Part print with two shaded views. Sizes in mm from the minimum x, y, z corner. Give positions to 0.01 mm unless a question says otherwise; leave off trailing zeros. Loops run counter-clockwise (first coordinate to the right, second up) from the corner with the lowest first, then second, coordinate; pieces in that order, holes last. Notation, with made-up numbers: M 41,-8 L 71,-8 A14 ccw 71,-4 Z; hole C -33,-30.5 d9. An arc over 180 degrees is marked long. Answer in a Markdown table with one row per item.
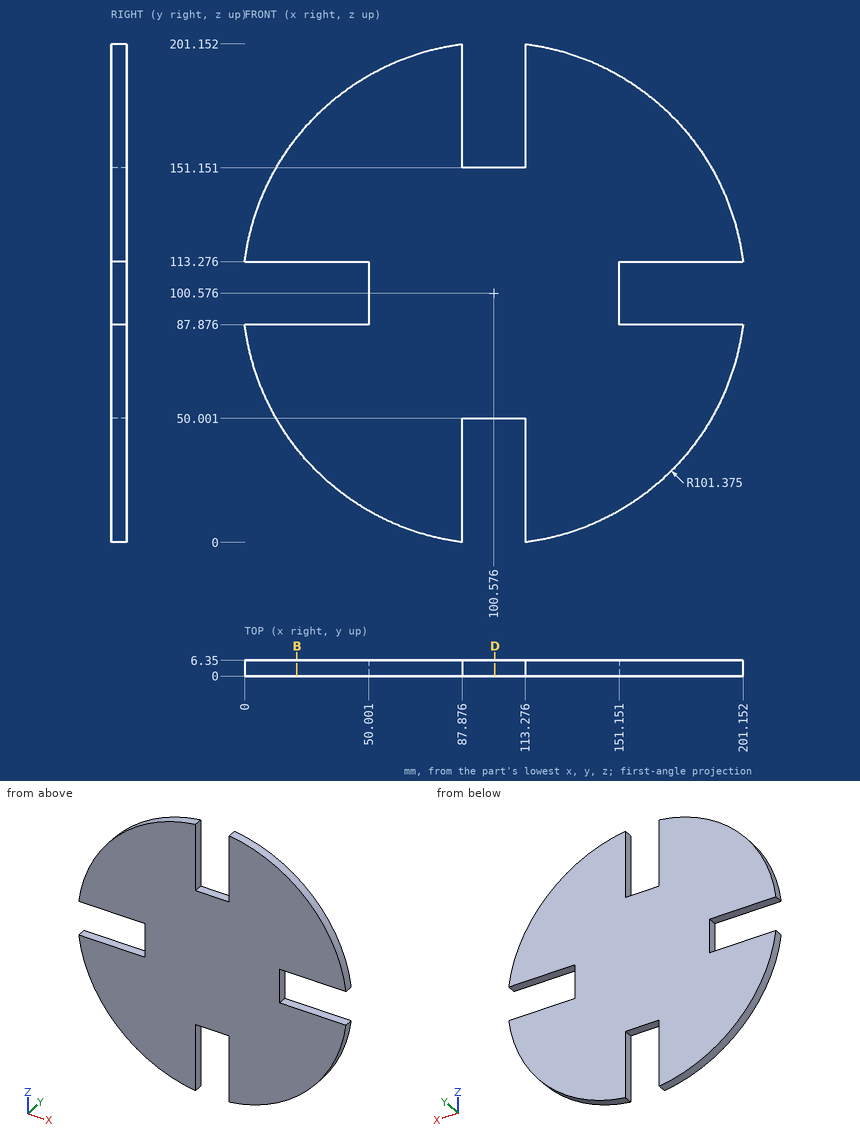
Q1. Saw through at D-D (x = 101). Give the cut face in (y, z).
Reported:
| item | result |
|---|---|
| outline | M 0,50 L 6.35,50 L 6.35,151.15 L 0,151.15 Z |
Q2. Saw through at B-B (x = 21). Give the cut face in (y, z).
Reported:
| item | result |
|---|---|
| outline | M 0,37.77 L 6.35,37.77 L 6.35,87.88 L 0,87.88 Z; M 0,113.28 L 6.35,113.28 L 6.35,163.38 L 0,163.38 Z |
Q3. Drop flat-ended pins along their axis: pin 1 (1.5 mm diameter, centred on x = 103.5, y = 1, fed in from -Z); pin 2 (1 mm diameter, centred on y = 4.5, z = 166.5, fed in from -X); pin 3 (3 mm diameter, centred on x = 17.5, y = 2.5, fed in from +Z). Give the stop position or say it passes through.
Reported:
| item | result |
|---|---|
| pin 1 | z = 50 |
| pin 2 | x = 23.14 |
| pin 3 | z = 160.76 |
Q4. Probe probe 1 along X at (y, z) = (1.75, 93); probe 2 along X at (y, z) = (2.5, 168) (1 decimal); probe 3 along Z at (x, y) = (28.5, 5.25) (1 decimal). List the from-to ranges inside material, lowest first.
Reported:
| item | result |
|---|---|
| probe 1 | 50 to 151.15 |
| probe 2 | 24.9 to 87.9, 113.3 to 176.3 |
| probe 3 | 29.3 to 87.9, 113.3 to 171.9 |
